The figure shows three views and two pictorial views of one solid part (mm, origin at its lowest corner). Answer the questions. Coordinates: 2 decimals unless noted, no trailing zeros. Write each loop counter-clockwise with the first axis right and the second up, starting at its lowest first coordinate (ties: lowest second). Pieces come first, ordered by that corner, then holes.
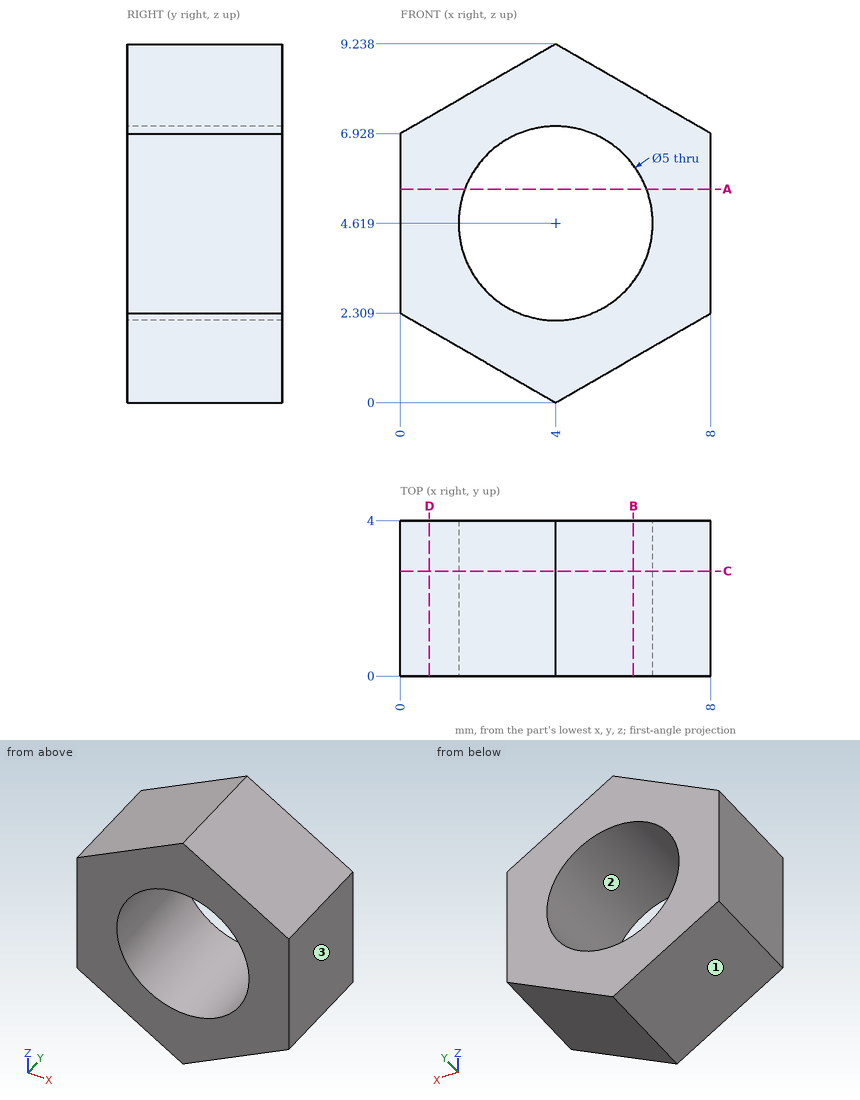
1. Section B-B on x = 6 is taken. Give the vertices of the cut face in (y, z) (1 decimal), then the cut area to 3 significant figures.
Results found:
outline: (0, 1.2) - (4, 1.2) - (4, 3.1) - (0, 3.1) - close; (0, 6.1) - (4, 6.1) - (4, 8.1) - (0, 8.1) - close
area: 15.7 mm2
2. Find the intervals of material crossed by L1, parallel to Z at x = 4.25, y = 2.1 (1 decimal); L2, parallel to Z at x = 5, y = 1.6; L3, parallel to X at y = 3.05, z = 4.75, in increasing order.
Results found:
L1: z = 0.1 to 2.1, 7.1 to 9.1
L2: z = 0.58 to 2.33, 6.91 to 8.66
L3: x = 0 to 1.5, 6.5 to 8
3. Section D-D on x = 0.75 is taken. Give the vertices of the cut face in (y, z).
Results found:
outline: (0, 1.88) - (4, 1.88) - (4, 7.36) - (0, 7.36) - close
4. For a pull along Z with two mould halves and no side action, classify the marked faces 1, 2 and 3 as pulls with the +Z half, pulls with the -Z half, needs draft (parallel to the pull), parting line crosses it, or undercut.
Results found:
face 1: pulls with the -Z half
face 2: undercut
face 3: needs draft
5. Section A-A on z = 5.5 is taken. Give the vertices of the cut face in (x, y), then the cut area to 3 significant figures.
Results found:
outline: (0, 0) - (1.66, 0) - (1.66, 4) - (0, 4) - close; (6.34, 0) - (8, 0) - (8, 4) - (6.34, 4) - close
area: 13.3 mm2
6. Flat-ended cylindrical pins translate along their axes: P1, Ø1.5, axis at x = 3.5, z = 5.5, coming from the +Y side; P2, Ø1, axis at x = 1.5, y = 2, coming from the -Z side (1 decimal); P3, Ø1.5, axis at y = 0.5, z = 8, coming from the -X side (1 decimal). Find the tip coordinate at first contact, or state that the pin passes through.
Results found:
P1: passes through
P2: stops at z = 1.2
P3: stops at x = 0.6
7. Section C-C on y = 2.7 is taken. Give the vertices of the cut face in (x, z).
Results found:
outline: (0, 2.31) - (4, 0) - (8, 2.31) - (8, 6.93) - (4, 9.24) - (0, 6.93) - close; hole circle Ø5 at (4, 4.62)
